Build history of the part. All positions in model axes, mm. Round coordinates to 2 decimals unless told otherwise and drop trailing zeros. Write each loop counter-clockwise with the first axis right and the second up, starting at its lowest first coordinate (ties: lowest second). Pieces come first, ordered by that corner, then holes. Notation, with made-up numbers: (85, 60) -> (138, 60) arc R24 ccw to (138, 98) -> close; hole circle Ø8 at (10.5, 62.25). An arc over 180 degrees is marked (long way). Return JSON: item names as keys, results as strings.
from build123d import *

# Parameters (mm, degrees)
F2_R     = 1.5
F3_DEPTH = 20.001
F4_W     = 1
F4_H     = 20.408089
F5_DEPTH = 25


with BuildPart() as f1:
    # F0 (on Top) → F1 (revolve)
    with BuildSketch(Plane.XY):
        Polygon((-10, 10), (-20, 20), (-21.414214, 18.585786), (-10, 7.171573), (-9, 0), (-5, 0), (-5, 10), align=None)
    revolve(axis=Axis((0, -1.348249, 0), (0, -1, 0)))

    # F2 (on face) → F3 (cut, through all)
    with BuildSketch(Plane.XZ):
        with Locations((0, 7)):
            Circle(F2_R)
    extrude(amount=-F3_DEPTH, mode=Mode.SUBTRACT)

    # F4 (on face) → F5 (cut)
    with BuildSketch(Plane.XZ):
        with Locations((0, -10.204045)):
            Rectangle(F4_W, F4_H)
    extrude(amount=-F5_DEPTH, mode=Mode.SUBTRACT)


solid = f1.part
Q1. Saw through at A-A on y = 4.25. List the corners of the cut face in (x, z), then the cut area to 3 significant figures.
Verdict:
{"outline": "(-0.5, -9.58) -> (-0.5, -4.97) arc R5 cw (long way) to (0.5, -4.97) -> (0.5, -9.58) arc R9.59 ccw (long way) to start; hole circle Ø3 at (0, 7)", "area": "199 mm²"}
Q2. Wall check: L1, parallel to X at y = 13.5, z = -4; L2, parallel to X at y = 10.75, z = -5; L3, parallel to Z at x = 0, y = 5.75. Give the ranges that are in metal, low to high.
Verdict:
{"L1": "x = -15.83 to -12.89, 12.89 to 15.83", "L2": "x = -12.62 to -9.52, 9.52 to 12.62", "L3": "z = 5 to 5.5, 8.5 to 9.8"}
Q3. Pin check, flat tips, straight feed: pin 1 Ø22 at (x, z) = (0, -0.5) entering from +Y; pin 2 Ø2 at (x, y) = (0.5, 16) entering from -Z; pin 3 Ø12 at (x, y) = (3.5, 9) entering from -Z. Stop position of each tip, or through.
Verdict:
{"pin 1": "stops at y = 11.5", "pin 2": "stops at z = -19.82", "pin 3": "stops at z = -17.57"}
Q4. Two-plate mould, pull along Z, no slides. Class faces 1 (the flat face through (-4, 0, 4)), 2 (the flat face through (2, 10, -5)), 3 (the conical face through (8.38, 7.73, 6.42)): +Z half, -Z half, draft (parallel to the pull), parting line (faces both ways), or undercut.
Verdict:
{"face 1": "draft", "face 2": "undercut", "face 3": "parting line"}
